The listing builds one solid part. Answer for the finished solid, in the listing's coordinates (mm). A direction names the side the tool comes from. Round coordinates to 2 decimals unless told otherwise and drop trailing zeros. Write each loop counter-clockwise with the first axis right and the second up, starting at its lowest first coordinate (ties: lowest second). Pieces come first, ordered by that corner, then holes.
from build123d import *

# Parameters (mm, degrees)
SKETCH2_R          = 6.35
CUT_EXTRUDE1_DEPTH = 106.839139341
CIRPATTERN1_COUNT  = 4


with BuildPart() as part:
    # Sketch1 → Revolve1 (revolve)
    with BuildSketch(Plane.XY, mode=Mode.PRIVATE) as revolve1_sk:
        with BuildLine():
            Line((-55.118, 19.05), (0, 19.05))
            Line((0, 19.05), (0, 69.85))
            Line((0, 69.85), (-12.8016, 69.85))
            ThreePointArc((-12.8016, 69.85), (-17.291728061, 67.990128061), (-19.1516, 63.5))
            Line((-19.1516, 63.5), (-19.1516, 41.275))
            ThreePointArc((-19.1516, 41.275), (-21.011471939, 36.784871939), (-25.5016, 34.925))
            Line((-25.5016, 34.925), (-50.8, 34.925))
            ThreePointArc((-50.8, 34.925), (-55.290128061, 33.065128061), (-57.15, 28.575))
            Line((-57.15, 28.575), (-57.15, 21.082))
            Line((-57.15, 21.082), (-55.118, 19.05))
        make_face()
    revolve(revolve1_sk.sketch.rotate(Axis((-117.274050633, 0, 0), (1, 0, 0)), 180), axis=Axis((-117.274050633, 0, 0), (1, 0, 0)))

    # Sketch2 → Cut-Extrude1 (cut, through all)
    with BuildSketch(Plane.ZY.offset(19.1516)):
        with Locations(Location((0, 53.975, 0), (0, 0, 270))):
            Circle(SKETCH2_R)
    cut_extrude1 = extrude(amount=-CUT_EXTRUDE1_DEPTH, mode=Mode.SUBTRACT)

    # CirPattern1: Cut-Extrude1 ×4 about axis
    cirpattern1_axis = Axis((0, 0, 0), (1, 0, 0))
    for i in range(1, CIRPATTERN1_COUNT):
        add(cut_extrude1.rotate(cirpattern1_axis, i * 360 / CIRPATTERN1_COUNT), mode=Mode.SUBTRACT)


solid = part.part
1. Given pin 1 (3 mm diameter, centred on x = -24, z = -8, fed in from +Y); pin 2 (1.5 mm diameter, centred on x = -51, z = -5.5, fed in from +Y); pin 3 (12 mm diameter, centred on y = -50.5, z = 27, fed in from +X); pin 4 (6 mm diameter, centred on x = -28, y = -31, fed in from -Z), each flat-ended and moving along its own axis, determine where each tip first touches the part or whether it passes through.
Geometry says:
pin 1: stops at y = 34.84
pin 2: stops at y = 34.6
pin 3: stops at x = 0
pin 4: stops at z = -20.87
2. Section D-D on x = -7.5 is taken. Determine the outline of the cut face in (y, z) (3 decimals), plus the area to 3 significant figures.
Geometry says:
outline: circle Ø139.7 at (0, 0); hole circle Ø12.7 at (-53.975, 0); hole circle Ø38.1 at (0, 0); hole circle Ø12.7 at (0, -53.975); hole circle Ø12.7 at (0, 53.975); hole circle Ø12.7 at (53.975, 0)
area: 13,700 mm2
3. Straight lines are drawn through the part: line 1 along Y through (x, z) = (-14.5, 3); line 2 along Z through (x, y) = (-28, 0) (3 decimals); line 3 along X through (y, z) = (36, -47.5). For each, find the intervals that lie inside material, in ascending order.
Geometry says:
line 1: y = -69.55 to -59.57, -48.38 to -18.81, 18.81 to 48.38, 59.57 to 69.55
line 2: z = -34.925 to -19.05, 19.05 to 34.925
line 3: x = -19.15 to 0
4. For a pull along Y with two mould halves and no side action, classify faces 3 (the face through (-9.71, 3.864, 59.014)), 4 (the face through (-9.71, 59.014, -3.864)), 5 (the face through (-38.328, 7.571, 34.094)), 6 (the face through (-57.15, 13, 17)) as released by +Y, released by -Y, zero draft, split by the parting line, or undercut.
Geometry says:
face 3: undercut
face 4: undercut
face 5: split by the parting line
face 6: zero draft
5. Section C-C on x = -31.5 is taken. Determine the outline of the cut face in (y, z) (3 decimals).
Geometry says:
outline: circle Ø69.85 at (0, 0); hole circle Ø38.1 at (0, 0)
6. A tool of negligible diameter and unlimited length cuts with its end or side. For faces 1 (the face through (-27.173, 4.13, 18.597)), 2 (the face through (-19.152, 0.89, 41.44)), from which of +Z, -Z, +X, -X, +Y, -Y can it reach the whole face along a straight path? Write none if from no direction.
Geometry says:
face 1: +X, -X
face 2: -X
7. Section A-A on y = 0 is taken. Determine the outline of the cut face in (x, z) (3 decimals).
Geometry says:
outline: (-57.15, -28.575) arc R6.35 ccw to (-50.8, -34.925) - (-25.502, -34.925) arc R6.35 cw to (-19.152, -41.275) - (-19.152, -47.625) - (0, -47.625) - (0, -19.05) - (-55.118, -19.05) - (-57.15, -21.082) - close; (-57.15, 21.082) - (-55.118, 19.05) - (0, 19.05) - (0, 47.625) - (-19.152, 47.625) - (-19.152, 41.275) arc R6.35 cw to (-25.502, 34.925) - (-50.8, 34.925) arc R6.35 ccw to (-57.15, 28.575) - close; (-19.152, -63.5) arc R6.35 ccw to (-12.802, -69.85) - (0, -69.85) - (0, -60.325) - (-19.152, -60.325) - close; (-19.152, 60.325) - (0, 60.325) - (0, 69.85) - (-12.802, 69.85) arc R6.35 ccw to (-19.152, 63.5) - close
